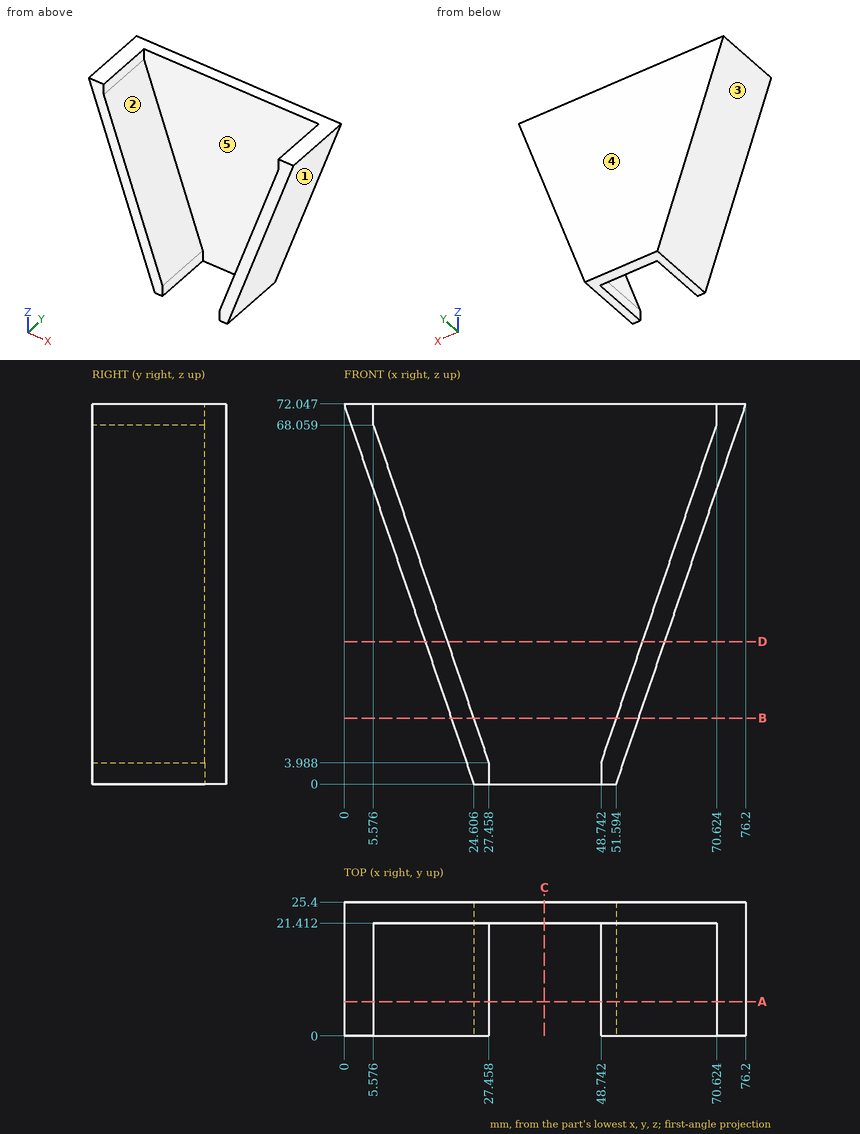
The figure shows three views and two pictorial views of one solid part (mm, origin at its lowest corner). Answer the questions. A direction names the side the tool comes from. Round coordinates to 2 decimals unless told otherwise and drop trailing zeros. Write each loop counter-clockwise with the first axis right and the second up, starting at its lowest first coordinate (ties: lowest second). Pieces come first, ordered by that corner, then holes. Notation, with made-up numbers: (3, -11.5) - (16, -11.5) arc R16 cw to (16, -5.5) - close; hole circle Ø7 at (3.25, 69.25). An arc over 180 degrees is marked (long way). One line per question, with ' | ' between items. Start each with the question number.
1. For the marked faces 1 and 2, determine the directions among +Z, -Z, +X, -X, +Y, -Y from which every point of the face is accessible in a straight line to the end or side of a thin tool.
2. For a pull along X with two mould halves and no side action, classify the marked faces 3, 4 and 5 as +X half, -X half, draft (parallel to the pull), parting line (faces both ways), or undercut.
3. Section B-B (z = 12.5) is taken. Determine the outline of the cut face in (x, y).
4. Find the intervals of material crossed by probe 1 along X at (y, z) = (9.25, 24); probe 2 along Y at (x, z) = (50, 43); probe 3 along X at (y, z) = (4, 53) (1 decimal), in increasing order. Write a range as [from, to].
5. Section C-C (x = 38) is taken. Determine the outline of the cut face in (y, z), and give its area (3 significant figures).
6. Section D-D (z = 27) is taken. Determine the outline of the cut face in (x, y) (1 decimal), and give its area (3 significant figures).
7. Each of these flat-tipped pins is pushed along its axis until it touches: pin 1 (3 mm diameter, centred on y = 11.5, z = 3, fed in from -X); pin 2 (4 mm diameter, centred on y = 20.5, z = 45, fed in from -X); pin 3 (2 mm diameter, centred on y = 13, z = 19, fed in from -X); pin 4 (5 mm diameter, centred on x = 47, y = 20.5, fed in from +Z). Where does it stop, or does it pass through?
8. Section A-A (y = 6.5) is taken. Determine the outline of the cut face in (x, z), and give its area (3 significant figures).
Filled in:
1) face 1: -Z, +X, +Y, -Y | face 2: +Z, -Y
2) face 3: -X half | face 4: draft | face 5: undercut
3) outline: (20.34, 0) - (24.55, 0) - (24.55, 21.41) - (51.65, 21.41) - (51.65, 0) - (55.86, 0) - (55.86, 25.4) - (20.34, 25.4) - close
4) probe 1: [16.41, 20.62], [55.58, 59.79] | probe 2: [21.41, 25.4] | probe 3: [6.5, 10.7], [65.5, 69.7]
5) outline: (21.41, 0) - (25.4, 0) - (25.4, 72.05) - (21.41, 72.05) - close | area: 287 mm²
6) outline: (15.4, 0) - (19.6, 0) - (19.6, 21.4) - (56.6, 21.4) - (56.6, 0) - (60.8, 0) - (60.8, 25.4) - (15.4, 25.4) - close | area: 362 mm²
7) pin 1: x = 23.07 | pin 2: x = 8.55 | pin 3: x = 17.78 | pin 4: z = 72.05
8) outline: (0, 72.05) - (24.61, 0) - (27.46, 0) - (27.46, 3.99) - (5.58, 68.06) - (5.58, 72.05) - close; (48.74, 0) - (51.59, 0) - (76.2, 72.05) - (70.62, 72.05) - (70.62, 68.06) - (48.74, 3.99) - close | area: 607 mm²
